The model under review builds one solid part; all positions refer to its coordinate system, in mm. A direction names the side the tool comes from. Coordinates: 2 decimals unless noted, no trailing zeros. Write each loop counter-clockwise with the first axis right and the second up, starting at its lowest first coordinate (ties: lowest second). Pieces come first, ordered by that corner, then holes. Notation, with made-up numbers: (54, -14.75) - (98, -14.75) arc R17 cw to (98, 18.25) - close; hole circle Ø3 at (23, -33.5). An arc over 180 degrees is marked (long way). Return JSON: item names as keys, results as strings. Group by question number.
(1) Draft analysis for pull direction Y (two halves, no side actions). For faces 1 (the face through (-0.54, -2.44, -5.67)), 2 (the face through (-1.2, 1.2, 8)), 3 (the face through (-1.5, 0.07, -1.86)), state which applies: released by +Y, released by -Y, zero draft, split by the parting line, or undercut.
(2) For pin 1 Ø1.5 at (y, z) = (-1.5, -7.5) entering from -X; pin 2 Ø5 at (y, z) = (2, -4) entering from -X; pin 3 Ø4 at (x, y) = (-3.5, -3) entering from -Z, all flat-tipped, find the tip position at first contact; note any pin that passes through.
(3) We need section C-C on z = 6. State the section outline as (x, y) points, then the cut area to 3 significant figures.
(4) To check wall thickness, follow L1, parallel to Y at x = 0, z = 5.5; L2, parallel to Z at x = 1, y = -3; L3, parallel to Y at x = -1, z = -3. State the ranges of each line that lie inside material, in increasing order. Write a range as from..to.
(5) We need section A-A on x = 0. State the section outline as (y, z) points, then the cut area to 3 significant figures.
(6) Tool access review of faces 4 (the face through (-1.08, 4.88, 3.94)), 5 (the face through (2, -2, 0)): name each direction out of +Z, -Z, +X, -X, +Y, -Y from which nothing blocks a thin tool from reaching the whole face with its end or side.
(7) We need section D-D on y = -4. State the section outline as (x, z) points.
Autodesk Inventor part; units mm, degrees
ref_plane "YZ Plane" through (0, 0, 0) normal (1, 0, 0) x (0, 1, 0)
ref_plane "XZ Plane" through (0, 0, 0) normal (0, 1, 0) x (-1, 0, 0)
ref_plane "XY Plane" through (0, 0, 0) normal (0, 0, 1) x (1, 0, 0)
sketch "Sketch1" plane through (0, 0, 0) normal (0, 0, 1) x (1, 0, 0)
  circle A0 centre (0, 0) radius 5
  circle A1 centre (0, 0) radius 2.5
  circle A2 centre (0, 0) radius 1.5
  dimension "d0" = 10
  dimension "d1" = 5
  dimension "d7" = 3
extrude "Extrusion1" add sketch "Sketch1" along normal blind 8 contours A0 | A1
extrude "Extrusion2" add sketch "Sketch1" against normal blind 12 contours A1
fillet "Fillet1" radius 0.5 1 edges at (-2.5, 0, -12)
properties part number "Tubing_Male_Connector"
Ans:
{
 "1": {"face 1": "split by the parting line", "face 2": "zero draft", "face 3": "undercut"},
 "2": {"pin 1": "x = -2.38", "pin 2": "x = -2.5", "pin 3": "z = 0"},
 "3": {"outline": "circle Ø10 at (0, 0); hole circle Ø3 at (0, 0)", "area": "71.5 mm²"},
 "4": {"L1": "-5..-1.5, 1.5..5", "L2": "0..8", "L3": "-2.29..-1.12, 1.12..2.29"},
 "5": {"outline": "(-5, 0) - (-2.5, 0) - (-2.5, -11.5) arc R0.5 ccw to (-2, -12) - (-1.5, -12) - (-1.5, 8) - (-5, 8) - close; (1.5, -12) - (2, -12) arc R0.5 ccw to (2.5, -11.5) - (2.5, 0) - (5, 0) - (5, 8) - (1.5, 8) - close", "area": "79.9 mm²"},
 "6": {"face 4": "+Z, -Z", "face 5": "-Z"},
 "7": {"outline": "(-3, 0) - (3, 0) - (3, 8) - (-3, 8) - close"}
}
